CAD build for the part. Positions are in the model's coordinates, mm. A direction names the side the tool comes from. Coordinates: 2 decimals unless noted, no trailing zeros. Write each loop counter-clockwise with the first axis right and the second up, starting at its lowest first coordinate (ties: lowest second). Pieces come first, ordered by that corner, then holes. Notation, with made-up numbers: (-13.5, -16.5) -> (42.5, -16.5) arc R24 cw to (42.5, 16.5) -> close; hole circle Ø8 at (3, -19). An arc over 180 degrees is marked (long way). Answer as CSV lines item,"result". Start each with the question number.
```python
from build123d import *

# Parameters (mm, degrees)
F0_W     = 101.6
F0_H     = 76.2
F0_R     = 3.9624
F0_W_2   = 12.7
F0_H_2   = 63.5
F1_DEPTH = 15.875
F2_DEPTH = 66.675
F3_W     = 6.35
F3_H     = 76.2
F4_DEPTH = 5.08
F5_R     = 12.7
F6_DEPTH = 25.4
F7_R     = 5.08


with BuildPart() as f1:
    # F0 (on Top) → F1 (new body)
    with BuildSketch(Plane.XY):
        Rectangle(F0_W, F0_H)
        with Locations((-34.163, -21.463)):
            Circle(F0_R, mode=Mode.SUBTRACT)
        Rectangle(F0_W_2, F0_H_2, mode=Mode.SUBTRACT)
        with Locations((-34.163, 21.463)):
            Circle(F0_R, mode=Mode.SUBTRACT)
    extrude(amount=-F1_DEPTH)

    # F0 (on Top) → F2 (join)
    with BuildSketch(Plane.XY):
        Rectangle(F0_W_2, F0_H_2)
    extrude(amount=-F2_DEPTH)

    # F3 (on face) → F4 (cut)
    with BuildSketch(Plane.XY):
        with Locations((25.4, 0)):
            Rectangle(F3_W, F3_H)
    extrude(amount=-F4_DEPTH, mode=Mode.SUBTRACT)

    # F5 (on face) → F6 (cut)
    with BuildSketch(Plane.YZ.offset(6.35)):
        with Locations((0, -41.275)):
            Circle(F5_R)
    extrude(amount=-F6_DEPTH, mode=Mode.SUBTRACT)

    # F7 (call 1 of 8: OpenCascade refuses the feature's edges together)
    f7_edges = [f1.edges().sort_by_distance(p)[0] for p in [
        (50.8, -38.1, -7.9375),
    ]]
    fillet(f7_edges, radius=F7_R)

    # F7#2 (call 2 of 8)
    f7_2_edges = [f1.edges().sort_by_distance(p)[0] for p in [
        (50.8, 38.1, -7.9375),
    ]]
    fillet(f7_2_edges, radius=F7_R)

    # F7#3 (call 3 of 8)
    f7_3_edges = [f1.edges().sort_by_distance(p)[0] for p in [
        (-50.8, 38.1, -7.9375),
    ]]
    fillet(f7_3_edges, radius=F7_R)

    # F7#4 (call 4 of 8)
    f7_4_edges = [f1.edges().sort_by_distance(p)[0] for p in [
        (-50.8, -38.1, -7.9375),
    ]]
    fillet(f7_4_edges, radius=F7_R)

    # F7#5 (call 5 of 8)
    f7_5_edges = [f1.edges().sort_by_distance(p)[0] for p in [
        (0, -31.75, -66.675),
    ]]
    fillet(f7_5_edges, radius=F7_R)

    # F7#6 (call 6 of 8)
    f7_6_edges = [f1.edges().sort_by_distance(p)[0] for p in [
        (0, 31.75, -66.675),
    ]]
    fillet(f7_6_edges, radius=F7_R)

    # F7#7 (call 7 of 8)
    f7_7_edges = [f1.edges().sort_by_distance(p)[0] for p in [
        (0, -31.75, -15.875),
    ]]
    fillet(f7_7_edges, radius=F7_R)

    # F7#8 (call 8 of 8)
    f7_8_edges = [f1.edges().sort_by_distance(p)[0] for p in [
        (0, 31.75, -15.875),
    ]]
    fillet(f7_8_edges, radius=F7_R)


solid = f1.part
```
1. Cut at C-C (x = 0.5). Give the cut face in (y, z) (3 decimals).
2. Tool access for faces 1 (the face through (0.09, -30.3, -65.15)), 2 (the face through (6.35, 8, -30)), 3 (the face through (0, 31.75, -41)): list every direction of +Z, -Z, +X, -X, +Y, -Y with a clear straight run to the whole face (end or side of a thin tool).
3. Cut at B-B (z = -52.5). Give the cut face in (x, y), then the cut area to 3 significant figures.
4. Cut at A-A (y = 0). Give the cut face in (x, z) (3 decimals).
5. Wall check: line 1 (Z direction, x = 2, y = 0) (3 decimals); line 2 (X direction, y = 18.5, z = -48.5); line 3 (Z direction, x = 24.5, y = 8.5) (3 decimals). Give the ranges that are in metal, low to high.
6. Flat gauge pins, fed straight in: P1, Ø14, axis at x = -3, z = -35.5, coming from the -Y side; P2, Ø14, axis at x = -1, z = -49.5, coming from the +Y side; P3, Ø3, axis at x = 27, y = -1, coming from the +Z side. Where does each tip first touch, or does it go through?
7. Cut at D-D (x = 25.5). Give the cut face in (y, z) (3 decimals).
8. Mould opens along Z. For faces 4 (the face through (0.1, -33.2, -17.4)), 5 (the face through (28.575, -1, -3)), 6 (the face through (0.089, -2.753, -53.673)), 7 (the face through (25, 1, -5.08)) say: pulls with the +Z half, pulls with the -Z half, needs draft (parallel to the pull), parting line crosses it, or undercut.
Geometry check:
1,outline,"(-38.1, -15.875) -> (-36.83, -15.875) arc R5.08 cw to (-31.75, -20.955) -> (-31.75, -61.595) arc R5.08 ccw to (-26.67, -66.675) -> (26.67, -66.675) arc R5.08 ccw to (31.75, -61.595) -> (31.75, -20.955) arc R5.08 cw to (36.83, -15.875) -> (38.1, -15.875) -> (38.1, 0) -> (-38.1, 0) -> close; hole circle Ø25.4 at (0, -41.275)"
2,face 1,"-Z, +X, -X, -Y"
2,face 2,"-Z, +X, +Y, -Y"
2,face 3,"-Z, +X, -X, +Y"
3,outline,"(-6.35, -31.75) -> (6.35, -31.75) -> (6.35, -5.94) -> (-6.35, -5.94) -> close; (-6.35, 5.94) -> (6.35, 5.94) -> (6.35, 31.75) -> (-6.35, 31.75) -> close"
3,area,"656 mm²"
4,outline,"(-50.8, -15.875) -> (-6.35, -15.875) -> (-6.35, -28.575) -> (6.35, -28.575) -> (6.35, -15.875) -> (50.8, -15.875) -> (50.8, 0) -> (28.575, 0) -> (28.575, -5.08) -> (22.225, -5.08) -> (22.225, 0) -> (-50.8, 0) -> close; (-6.35, -66.675) -> (6.35, -66.675) -> (6.35, -53.975) -> (-6.35, -53.975) -> close"
5,line 1,"-66.675 to -53.975, -28.575 to 0"
5,line 2,"-6.35 to 6.35"
5,line 3,"-15.875 to -5.08"
6,P1,"y = -31.75"
6,P2,"y = 31.75"
6,P3,"z = -5.08"
7,outline,"(-38.1, -15.875) -> (38.1, -15.875) -> (38.1, -5.08) -> (-38.1, -5.08) -> close"
8,face 4,"pulls with the -Z half"
8,face 5,"needs draft"
8,face 6,"undercut"
8,face 7,"pulls with the +Z half"
